Job drawing, mm, ordinate dimensions from the low corner. One solid piece. A direction names the side the tool comes from. Give positions to 0.01 mm unless a question says otherwise; leave off trailing zeros. Write each loop counter-clockwise with the first axis right and the second up, starting at its lowest first coordinate (ties: lowest second). Pieces come first, ordered by that corner, then holes. Notation, with made-up numbers: (27, 18.5) -> (66, 18.5) arc R27 cw to (66, 48.5) -> close; hole circle Ø10 at (-26, 88.25). An arc over 180 degrees is marked (long way). Put each result on its own line as item: value. Start each with the question number.
Item 1: Slice it at D-D, the plane x = 32.5. List the corners of the cut face in (y, z) (1 decimal).
Item 2: Tool access for the marked faces 1, 2, 3 and 4: list every direction of +Z, -Z, +X, -X, +Y, -Y with a clear straight run to the whole face (end or side of a thin tool).
Item 3: Drill centre lines: line 1 along Z through (x, y) = (27, 6.5) (1 decimal); line 2 along Z through (x, y) = (2.5, 4.5) (1 decimal). Where is each one in solid material? Low to high.
Item 4: Flat gauge pins, fed straight in: pin 1 Ø3 at (y, z) = (2, 21.5) entering from +X (1 decimal); pin 2 Ø1.9 at (x, y) = (4, 4) entering from +Z; pin 3 Ø5 at (x, y) = (22.5, 1) entering from +Z (1 decimal). Where does each tip first touch, or does it go through?
Item 5: Slice it at B-B, the plane x = 12.7. List the corners of the cut face in (y, z) (1 decimal).
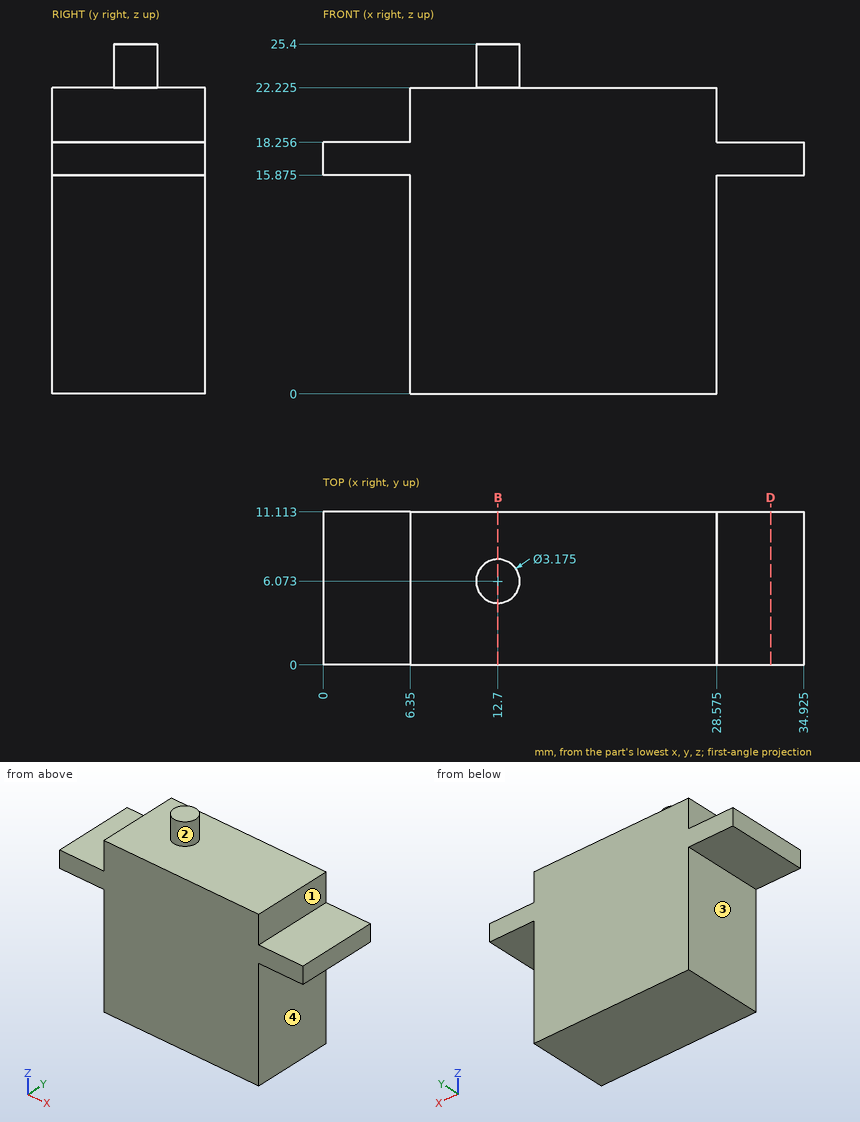
Values follow:
1. outline: (0, 15.9) -> (11.1, 15.9) -> (11.1, 18.3) -> (0, 18.3) -> close
2. face 1: +Z, +X, +Y, -Y
2. face 2: +Z
2. face 3: -Z, -X, +Y, -Y
2. face 4: -Z, +X, +Y, -Y
3. line 1: 0 to 22.2
3. line 2: 15.9 to 18.3
4. pin 1: x = 28.6
4. pin 2: z = 18.26
4. pin 3: z = 22.2
5. outline: (0, 0) -> (11.1, 0) -> (11.1, 22.2) -> (7.7, 22.2) -> (7.7, 25.4) -> (4.5, 25.4) -> (4.5, 22.2) -> (0, 22.2) -> close
